Input: part model. Units: mm. Frame: model coordinates. Round coordinates to 2 decimals unless told otherwise and drop trailing zeros. Write each loop counter-clockwise with the first axis right and the second up, starting at its lowest first coordinate (ties: lowest second). Pieces come first, ordered by that corner, then holes. Notation, with made-up numbers: (64, -26) - (75, -26) arc R11 cw to (75, -22) - close; hole circle Ø1 at (-20, 43.25). An arc over 180 degrees is marked (long way). Use one line per item in the form item = value.
```python
from build123d import *

# Parameters (mm, degrees)
SKETCH1_R                    = 1.5
SKETCH1_R_2                  = 2.2
SKETCH1_R_3                  = 2
SKETCH1_R_4                  = 4
BASE_FLANGE1_DEPTH           = 2
SKETCHED_START               = -20.5
SKETCHED_BEND1_DEPTH         = 41
SKETCHED_START_2             = -29
SKETCHED_BEND1_2_DEPTH       = 9
SKETCHED_START_3             = 20
SKETCHED_BEND1_3_DEPTH       = 9
SKETCHED_BEND1_4_DEPTH       = 41
SKETCHED_BEND1_5_DEPTH       = 9
SKETCHED_BEND1_6_DEPTH       = 9
SKETCHED_START_4             = -25
SKETCHED_BEND1_7_OUTLINE_R   = 1.5
SKETCHED_BEND1_7_OUTLINE_R_2 = 2.2
SKETCHED_BEND1_7_DEPTH       = 32
SKETCHED_START_5             = 5
SKETCHED_BEND1_8_DEPTH       = 2


with BuildPart() as part:
    # Base-Flange1: sheet metal written as solids
    # Sketch1 → Base-Flange1 (new body)
    with BuildSketch(Plane(origin=(0, 0, 0), x_dir=(1, 0, 0), z_dir=(0, 1, 0))):
        with BuildLine():
            Line((-27, 0), (-20.5, 0))
            Line((-20.5, 0), (-20.5, -27))
            ThreePointArc((-20.5, -27), (-19.914213562, -28.414213562), (-18.5, -29))
            Line((-18.5, -29), (18.5, -29))
            ThreePointArc((18.5, -29), (19.914213562, -28.414213562), (20.5, -27))
            Line((20.5, -27), (20.5, 0))
            Line((20.5, 0), (27, 0))
            ThreePointArc((27, 0), (28.414213562, 0.585786438), (29, 2))
            Line((29, 2), (29, 48))
            ThreePointArc((29, 48), (28.414213562, 49.414213562), (27, 50))
            Line((27, 50), (22, 50))
            ThreePointArc((22, 50), (20.585786438, 49.414213562), (20, 48))
            Line((20, 48), (20, 20))
            Line((20, 20), (18, 20))
            Line((18, 20), (18, 26))
            ThreePointArc((18, 26), (17.414213562, 27.414213562), (16, 28))
            Line((16, 28), (-16, 28))
            ThreePointArc((-16, 28), (-17.414213562, 27.414213562), (-18, 26))
            Line((-18, 26), (-18, 20))
            Line((-18, 20), (-20, 20))
            Line((-20, 20), (-20, 48))
            ThreePointArc((-20, 48), (-20.585786438, 49.414213562), (-22, 50))
            Line((-22, 50), (-27, 50))
            ThreePointArc((-27, 50), (-28.414213562, 49.414213562), (-29, 48))
            Line((-29, 48), (-29, 2))
            ThreePointArc((-29, 2), (-28.414213562, 0.585786438), (-27, 0))
        make_face()
        with Locations(Location((-17, -17.5, 0), (0, 0, 270))):
            Circle(SKETCH1_R, mode=Mode.SUBTRACT)
        with Locations(Location((-10, -17.5, 0), (0, 0, 270))):
            Circle(SKETCH1_R, mode=Mode.SUBTRACT)
        with Locations(Location((-10, -10.5, 0), (0, 0, 270))):
            Circle(SKETCH1_R, mode=Mode.SUBTRACT)
        with Locations(Location((-3, -17.5, 0), (0, 0, 270))):
            Circle(SKETCH1_R, mode=Mode.SUBTRACT)
        with Locations(Location((-10, -24.5, 0), (0, 0, 270))):
            Circle(SKETCH1_R, mode=Mode.SUBTRACT)
        with Locations(Location((24.4, 40.5, 0), (0, 0, 270))):
            Circle(SKETCH1_R_2, mode=Mode.SUBTRACT)
        with Locations(Location((24.4, 30.5, 0), (0, 0, 270))):
            Circle(SKETCH1_R_2, mode=Mode.SUBTRACT)
        with Locations(Location((-24.4, 30.5, 0), (0, 0, 90))):
            Circle(SKETCH1_R_2, mode=Mode.SUBTRACT)
        with Locations(Location((-24.4, 40.5, 0), (0, 0, 90))):
            Circle(SKETCH1_R_2, mode=Mode.SUBTRACT)
        with Locations(Location((24.4, 6, 0), (0, 0, 270))):
            Circle(SKETCH1_R_3, mode=Mode.SUBTRACT)
        with Locations(Location((24.4, 16, 0), (0, 0, 270))):
            Circle(SKETCH1_R_3, mode=Mode.SUBTRACT)
        with Locations(Location((-24.4, 16, 0), (0, 0, 90))):
            Circle(SKETCH1_R_3, mode=Mode.SUBTRACT)
        with Locations(Location((-24.4, 6, 0), (0, 0, 90))):
            Circle(SKETCH1_R_3, mode=Mode.SUBTRACT)
        with Locations(Location((0, -1, 0), (0, 0, 270))):
            Circle(SKETCH1_R, mode=Mode.SUBTRACT)
        with Locations(Location((0, 6.5, 0), (0, 0, 270))):
            Circle(SKETCH1_R_4, mode=Mode.SUBTRACT)
        with Locations(Location((-7.5, 6.5, 0), (0, 0, 270))):
            Circle(SKETCH1_R, mode=Mode.SUBTRACT)
        with Locations(Location((0, 14, 0), (0, 0, 270))):
            Circle(SKETCH1_R, mode=Mode.SUBTRACT)
        with Locations(Location((7.5, 6.5, 0), (0, 0, 270))):
            Circle(SKETCH1_R, mode=Mode.SUBTRACT)
        with Locations(Location((-3.5, 17.5, 0), (0, 0, 270))):
            Circle(SKETCH1_R, mode=Mode.SUBTRACT)
        with Locations(Location((-11, 17.5, 0), (0, 0, 270))):
            Circle(SKETCH1_R_4, mode=Mode.SUBTRACT)
        with Locations(Location((-11, 25, 0), (0, 0, 270))):
            Circle(SKETCH1_R, mode=Mode.SUBTRACT)
        with Locations(Location((-18.5, 17.5, 0), (0, 0, 270))):
            Circle(SKETCH1_R, mode=Mode.SUBTRACT)
        with Locations(Location((-11, 10, 0), (0, 0, 270))):
            Circle(SKETCH1_R, mode=Mode.SUBTRACT)
        with Locations(Location((3.5, 17.5, 0), (0, 0, 270))):
            Circle(SKETCH1_R, mode=Mode.SUBTRACT)
        with Locations(Location((11, 17.5, 0), (0, 0, 270))):
            Circle(SKETCH1_R_4, mode=Mode.SUBTRACT)
        with Locations(Location((11, 10, 0), (0, 0, 270))):
            Circle(SKETCH1_R, mode=Mode.SUBTRACT)
        with Locations(Location((18.5, 17.5, 0), (0, 0, 270))):
            Circle(SKETCH1_R, mode=Mode.SUBTRACT)
        with Locations(Location((11, 25, 0), (0, 0, 270))):
            Circle(SKETCH1_R, mode=Mode.SUBTRACT)
        with Locations(Location((10, -10.5, 0), (0, 0, 90))):
            Circle(SKETCH1_R, mode=Mode.SUBTRACT)
        with Locations(Location((10, -24.5, 0), (0, 0, 90))):
            Circle(SKETCH1_R, mode=Mode.SUBTRACT)
        with Locations(Location((3, -17.5, 0), (0, 0, 90))):
            Circle(SKETCH1_R, mode=Mode.SUBTRACT)
        with Locations(Location((10, -17.5, 0), (0, 0, 90))):
            Circle(SKETCH1_R, mode=Mode.SUBTRACT)
        with Locations(Location((17, -17.5, 0), (0, 0, 90))):
            Circle(SKETCH1_R, mode=Mode.SUBTRACT)
    extrude(amount=-BASE_FLANGE1_DEPTH)

    # Sketched Bend1: read off the stored shape, not the designer's step
    # Sketched Bend1 outline → Sketched Bend1 (cut)
    with BuildSketch(Plane.YZ.offset(SKETCHED_START)):
        with BuildLine():
            Line((-2, 29), (-2, 4.2634))
            ThreePointArc((-2, 4.2634), (-1.443395312, 5.917667209), (0, 6.899002398))
            Line((0, 6.899002398), (0, 29))
            Line((0, 29), (-2, 29))
        make_face()
    extrude(amount=SKETCHED_BEND1_DEPTH, mode=Mode.SUBTRACT)

    # Sketched Bend1 2 outline → Sketched Bend1 2 (cut)
    with BuildSketch(Plane.YZ.offset(SKETCHED_START_2)):
        with BuildLine():
            ThreePointArc((0, -24.899002398), (-1.443395312, -23.917667209), (-2, -22.2634))
            Line((-2, -22.2634), (-2, -50))
            Line((-2, -50), (0, -50))
            Line((0, -50), (0, -24.899002398))
        make_face()
    extrude(amount=SKETCHED_BEND1_2_DEPTH, mode=Mode.SUBTRACT)

    # Sketched Bend1 3 outline → Sketched Bend1 3 (cut)
    with BuildSketch(Plane.YZ.offset(SKETCHED_START_3)):
        with BuildLine():
            ThreePointArc((0, -24.899002398), (-1.443395312, -23.917667209), (-2, -22.2634))
            Line((-2, -22.2634), (-2, -50))
            Line((-2, -50), (0, -50))
            Line((0, -50), (0, -24.899002398))
        make_face()
    extrude(amount=SKETCHED_BEND1_3_DEPTH, mode=Mode.SUBTRACT)

    # Sketched Bend1 4 outline → Sketched Bend1 4 (add)
    with BuildSketch(Plane.YZ.offset(SKETCHED_START)):
        with BuildLine():
            ThreePointArc((0.7366, 7), (0.364854094, 6.974633029), (0, 6.899002398))
            Line((0, 6.899002398), (0, 4.2634))
            ThreePointArc((0, 4.2634), (0.215745145, 4.784254855), (0.7366, 5))
            Line((0.7366, 5), (22.745355099, 5))
            Line((22.745355099, 5), (22.745355099, 7))
            Line((22.745355099, 7), (0.7366, 7))
        make_face()
    extrude(amount=SKETCHED_BEND1_4_DEPTH)

    # Sketched Bend1 5 outline → Sketched Bend1 5 (add)
    with BuildSketch(Plane.YZ.offset(SKETCHED_START_2)):
        with BuildLine():
            Line((0, -22.2634), (0, -24.899002398))
            ThreePointArc((0, -24.899002398), (0.364854094, -24.974633029), (0.7366, -25))
            Line((0.7366, -25), (25.745355099, -25))
            Line((25.745355099, -25), (25.745355099, -23))
            Line((25.745355099, -23), (0.7366, -23))
            ThreePointArc((0.7366, -23), (0.215745145, -22.784254855), (0, -22.2634))
        make_face()
    extrude(amount=SKETCHED_BEND1_5_DEPTH)

    # Sketched Bend1 6 outline → Sketched Bend1 6 (add)
    with BuildSketch(Plane.YZ.offset(SKETCHED_START_3)):
        with BuildLine():
            Line((0, -22.2634), (0, -24.899002398))
            ThreePointArc((0, -24.899002398), (0.364854094, -24.974633029), (0.7366, -25))
            Line((0.7366, -25), (25.745355099, -25))
            Line((25.745355099, -25), (25.745355099, -23))
            Line((25.745355099, -23), (0.7366, -23))
            ThreePointArc((0.7366, -23), (0.215745145, -22.784254855), (0, -22.2634))
        make_face()
    extrude(amount=SKETCHED_BEND1_6_DEPTH)

    # Sketched Bend1 7 outline → Sketched Bend1 7 (cut)
    with BuildSketch(Plane.XY.offset(SKETCHED_START_4)):
        with BuildLine():
            ThreePointArc((-29, 23.745355099), (-28.414213562, 25.159568661), (-27, 25.745355099))
            Line((-27, 25.745355099), (-29, 25.745355099))
            Line((-29, 25.745355099), (-29, 23.745355099))
        make_face()
        with BuildLine():
            ThreePointArc((-22, 25.745355099), (-20.585786438, 25.159568661), (-20, 23.745355099))
            Line((-20, 23.745355099), (-20, 25.745355099))
            Line((-20, 25.745355099), (-22, 25.745355099))
        make_face()
        with BuildLine():
            Line((29, 25.745355099), (27, 25.745355099))
            ThreePointArc((27, 25.745355099), (28.414213562, 25.159568661), (29, 23.745355099))
            Line((29, 23.745355099), (29, 25.745355099))
        make_face()
        with BuildLine():
            Line((20, 25.745355099), (20, 23.745355099))
            ThreePointArc((20, 23.745355099), (20.585786438, 25.159568661), (22, 25.745355099))
            Line((22, 25.745355099), (20, 25.745355099))
        make_face()
        with BuildLine():
            Line((20, 22.745355099), (18.5, 22.745355099))
            ThreePointArc((18.5, 22.745355099), (19.322875656, 22.568230754), (20, 22.068230754))
            Line((20, 22.068230754), (20, 22.745355099))
        make_face()
        with BuildLine():
            Line((-20, 22.745355099), (-20, 22.068230754))
            ThreePointArc((-20, 22.068230754), (-19.322875656, 22.568230754), (-18.5, 22.745355099))
            Line((-18.5, 22.745355099), (-20, 22.745355099))
        make_face()
        with Locations((17, 11.245355099)):
            Circle(SKETCHED_BEND1_7_OUTLINE_R)
        with Locations((-10, 18.245355099)):
            Circle(SKETCHED_BEND1_7_OUTLINE_R)
        with Locations((-3, 11.245355099)):
            Circle(SKETCHED_BEND1_7_OUTLINE_R)
        with Locations((-10, 4.245355099)):
            Circle(SKETCHED_BEND1_7_OUTLINE_R)
        with Locations((-17, 11.245355099)):
            Circle(SKETCHED_BEND1_7_OUTLINE_R)
        with Locations((10, 11.245355099)):
            Circle(SKETCHED_BEND1_7_OUTLINE_R)
        with Locations((3, 11.245355099)):
            Circle(SKETCHED_BEND1_7_OUTLINE_R)
        with Locations((10, 18.245355099)):
            Circle(SKETCHED_BEND1_7_OUTLINE_R)
        with Locations((-10, 11.245355099)):
            Circle(SKETCHED_BEND1_7_OUTLINE_R)
        with Locations((10, 4.245355099)):
            Circle(SKETCHED_BEND1_7_OUTLINE_R)
        with Locations((24.4, 16.245355099)):
            Circle(SKETCHED_BEND1_7_OUTLINE_R_2)
        with Locations((24.4, 6.245355099)):
            Circle(SKETCHED_BEND1_7_OUTLINE_R_2)
        with Locations((-24.4, 6.245355099)):
            Circle(SKETCHED_BEND1_7_OUTLINE_R_2)
        with Locations((-24.4, 16.245355099)):
            Circle(SKETCHED_BEND1_7_OUTLINE_R_2)
    extrude(amount=SKETCHED_BEND1_7_DEPTH, mode=Mode.SUBTRACT)

    # Sketched Bend1 8 outline → Sketched Bend1 8 (cut)
    with BuildSketch(Plane.XY.offset(SKETCHED_START_5)):
        with BuildLine():
            Line((-20.5, 22.745355099), (-20.5, 20.745355099))
            ThreePointArc((-20.5, 20.745355099), (-20.370828693, 21.45246188), (-20, 22.068230754))
            Line((-20, 22.068230754), (-20, 22.745355099))
            Line((-20, 22.745355099), (-20.5, 22.745355099))
        make_face()
        with BuildLine():
            Line((20, 22.745355099), (20, 22.068230754))
            ThreePointArc((20, 22.068230754), (20.370828693, 21.45246188), (20.5, 20.745355099))
            Line((20.5, 20.745355099), (20.5, 22.745355099))
            Line((20.5, 22.745355099), (20, 22.745355099))
        make_face()
    extrude(amount=SKETCHED_BEND1_8_DEPTH, mode=Mode.SUBTRACT)


solid = part.part
```
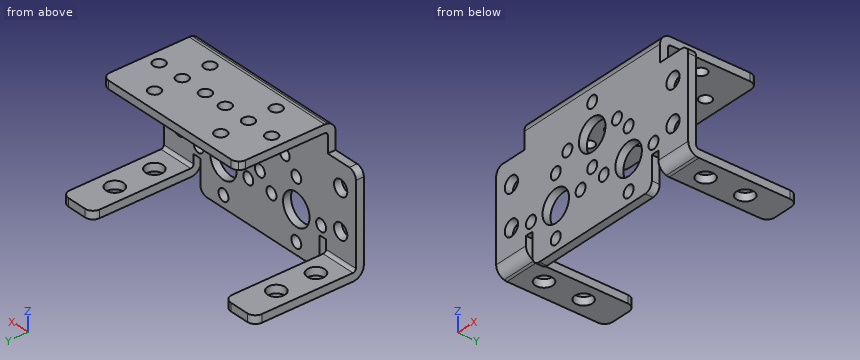
(1) Cut plane A-A on x = 0. Output: boundary loops of the cut face in (y, z), then the cut area to 3 significant figures.
Derived:
outline = (-2, -28) - (0, -28) - (0, -15.5) - (-2, -15.5) - close; (-2, -12.5) - (0, -12.5) - (0, -10.5) - (-2, -10.5) - close; (-2, -2.5) - (0, -2.5) - (0, -0.5) - (-2, -0.5) - close; (-2, 2.5) - (0, 2.5) - (0, 4.26) arc R0.74 cw to (0.74, 5) - (22.75, 5) - (22.75, 7) - (0.74, 7) arc R2.74 ccw to (-2, 4.26) - close
area = 86.0 mm^2
(2) First-contact query: pin 1 Ø2 at (x, z) = (-4, 0.5) entering from +Y; pin 2 Ø2.5 at (x, z) = (-24.4, -16) entering from -Y; pin 3 Ø4.5 at (x, y) = (23, 16.5) entering from +Z; pin 4 Ø4 at (x, y) = (10, 11.25) entering from -Z. Flat tips, straight axial feed; report the tip coordinate or a pass-through.
Derived:
pin_1 = 0
pin_2 = through
pin_3 = -23
pin_4 = 5
(3) Cut plane B-B on z = -7. Output: boundary loops of the cut face in (x, y).
Derived:
outline = (-29, -2) - (-26.13, -2) - (-26.13, 0) - (-29, 0) - close; (-22.67, -2) - (-8.91, -2) - (-8.91, 0) - (-22.67, 0) - close; (-6.09, -2) - (-3.97, -2) - (-3.97, 0) - (-6.09, 0) - close; (3.97, -2) - (6.09, -2) - (6.09, 0) - (3.97, 0) - close; (8.91, -2) - (22.67, -2) - (22.67, 0) - (8.91, 0) - close; (26.13, -2) - (29, -2) - (29, 0) - (26.13, 0) - close
(4) Material intervals for L1, parallel to X at y = -1.4, z = -6.5; L2, parallel to Y at x = 16.5, z = -5.5; L3, parallel to Z at x = 0, y = 17.25, sorted ascending.
Derived:
L1 = -29 to -26.34, -22.46 to -9, -6 to -4, 4 to 6, 9 to 22.46, 26.34 to 29
L2 = -2 to 0
L3 = 5 to 7
(5) Cut plane C-C on y = 12. Count the separate pieces of the cut face and the enclosed holes in it, then the cut area to 3 significant figures.
Derived:
separate_pieces = 9
enclosed_holes = 0
area = 86.9 mm^2
